Geometry check sheet. Reference: drawing and pictorial views, mm from the part's lowest x, y, z. A direction names the side the tool comes from. Give positions to 0.01 mm unless a question says otherwise; leave off trailing zeros. Order: outer loops, then holes, each group sorted by start corner. A loop starts at its lowest first (then second) coordinate and runs counter-clockwise, first axis right, second up. Notation, with made-up numbers: (-15.75, 8.5) - (21.25, 8.5) arc R9 ccw to (21.25, 25.5) - close; hole circle Ø2 at (-36.5, 81). An arc over 180 degrees is marked (long way). Answer in a Markdown table with one row per item.
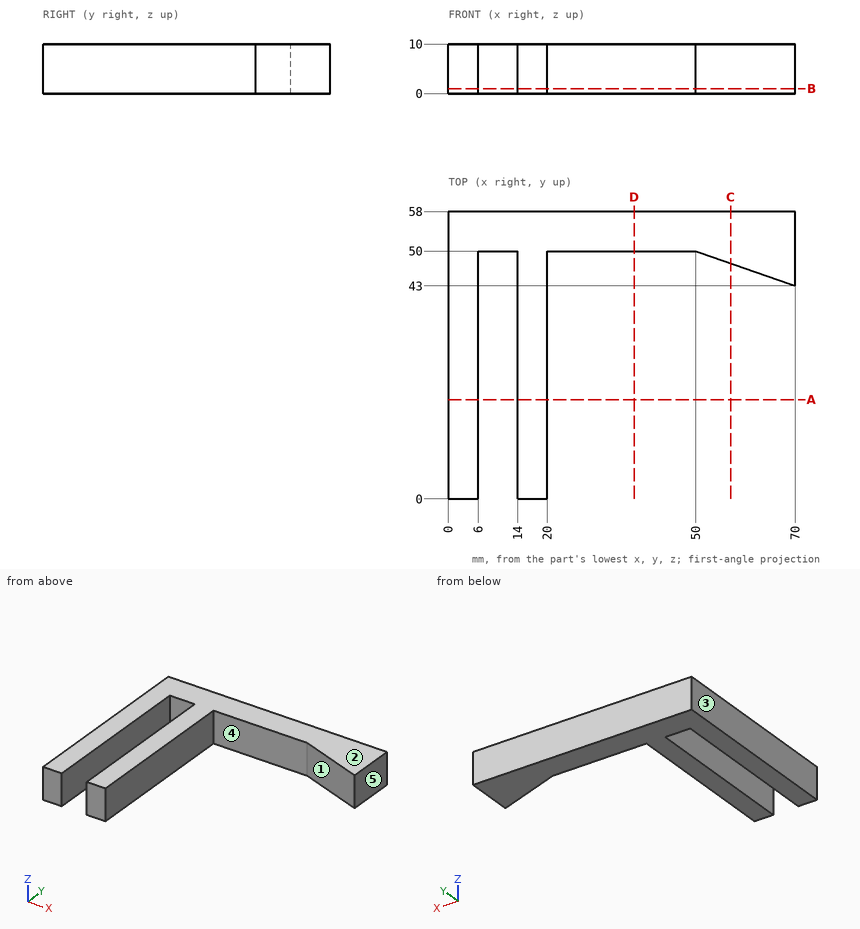
(1) Mould release check, pull along X, two halves, no side actions. Record for the marked faces 1, 2 and 3: pulls with the +X half, pulls with the -X half, needs draft (parallel to the pull), parting line crosses it, or undercut.
Geometry says:
| item | result |
|---|---|
| face 1 | undercut |
| face 2 | needs draft |
| face 3 | pulls with the -X half |
(2) Cross-section at A-A, the plane y = 20. Record the cut outline in (x, z).
Geometry says:
| item | result |
|---|---|
| outline | (0, 0) - (6, 0) - (6, 10) - (0, 10) - close; (14, 0) - (20, 0) - (20, 10) - (14, 10) - close |
(3) Access from +Z, -Z, +X, -X, +Y, -Y to the whole of each face (thin tool, end or side, straight path). Record for the marked faces 4 and 5.
Geometry says:
| item | result |
|---|---|
| face 4 | +Z, -Z, -Y |
| face 5 | +Z, -Z, +X, +Y, -Y |
(4) Cross-section at C-C, the plane x = 57. Record the cut outline in (y, z).
Geometry says:
| item | result |
|---|---|
| outline | (47.55, 0) - (58, 0) - (58, 10) - (47.55, 10) - close |
(5) Cross-section at B-B, the plane z = 1. Record the cut outline in (x, y).
Geometry says:
| item | result |
|---|---|
| outline | (0, 0) - (6, 0) - (6, 50) - (14, 50) - (14, 0) - (20, 0) - (20, 50) - (50, 50) - (70, 43) - (70, 58) - (0, 58) - close |
(6) Cross-section at D-D, the plane x = 37.5. Record the cut outline in (y, z).
Geometry says:
| item | result |
|---|---|
| outline | (50, 0) - (58, 0) - (58, 10) - (50, 10) - close |
(7) Thickness scan on L1, parallel to X at y = 41, z = 5.75; L2, parallel to Y at x = 48, z = 9.75; L3, parallel to Y at x = 60, z = 6. Record the ranges inside material, lowest first.
Geometry says:
| item | result |
|---|---|
| L1 | 0 to 6, 14 to 20 |
| L2 | 50 to 58 |
| L3 | 46.5 to 58 |
(8) Gauge pin test, flat ends, axial feed: P1, Ø5, axis at y = 18, z = 6, coming from the +X side; P2, Ø1.5, axis at x = 54.5, z = 7.5, coming from the -Y side; P3, Ø5, axis at x = 39.5, z = 7.5, coming from the -Y side. Record the tip position at first contact, or that the pin passes through.
Geometry says:
| item | result |
|---|---|
| P1 | x = 20 |
| P2 | y = 48.16 |
| P3 | y = 50 |
